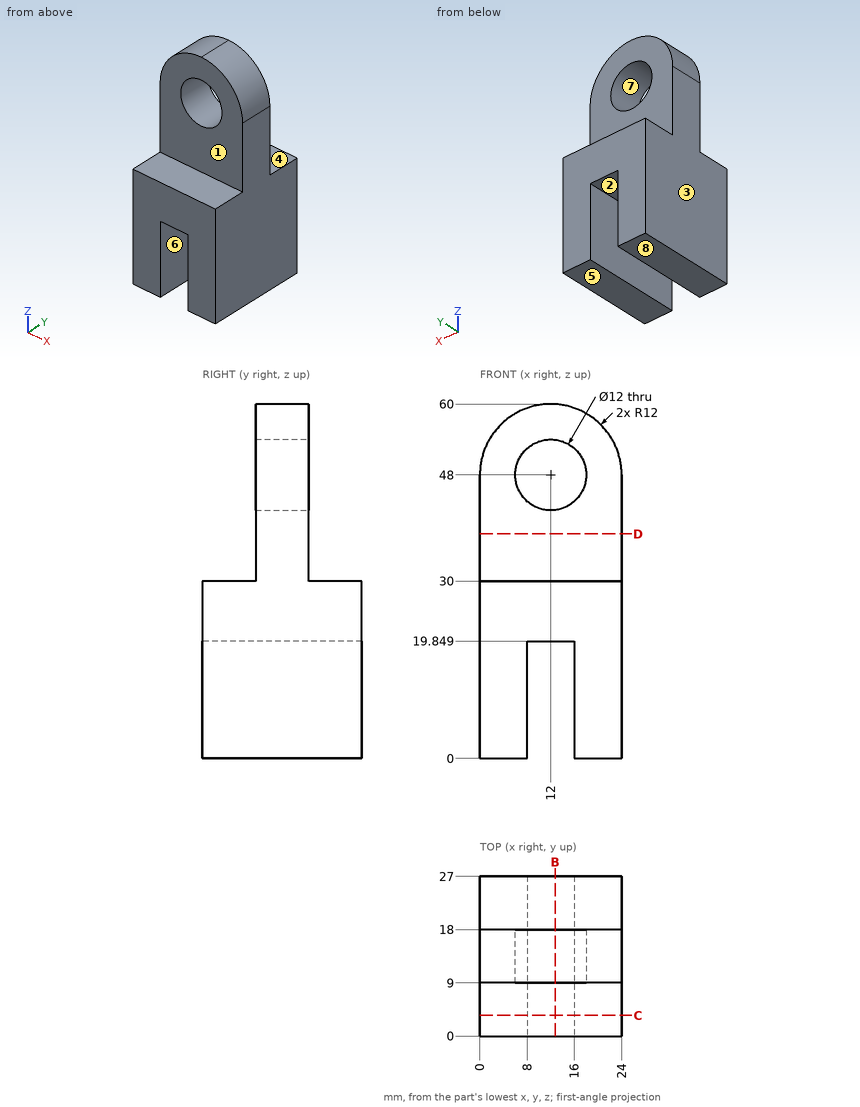
Design review of the part shown in the three views and the two pictorial views. Dimensions are in mm from the part's minimum x, y and z. A direction names the side the tool comes from. Give positions to 0.01 mm unless a question says otherwise; leave off trailing zeros. Write each loop counter-clockwise with the first axis right and the second up, starting at its lowest first coordinate (ties: lowest second). Pieces come first, ordered by that corner, then holes. Notation, with made-up numbers: (29.5, 73.5) -> (37.5, 73.5) arc R23 cw to (37.5, 86.5) -> close; hole circle Ø10 at (47, 35.5). An arc over 180 degrees is marked (long way). Answer in a Markdown table with one row per item.
1) For L1, parallel to Z at x = 12.25, y = 17.75 (1 decimal); L2, parallel to X at y = 12.25, z = 48; L3, parallel to X at y = 16.75, z = 16, list the stretches that pass through material, from the lowest coordinate up. Write a range as [from, to].
Worked answers:
| item | result |
|---|---|
| L1 | [19.8, 42], [54, 60] |
| L2 | [0, 6], [18, 24] |
| L3 | [0, 8], [16, 24] |
2) Mouldability with a two-part tool opening along Z and no side actions: class the marked faces 6, 7 and 8 as +Z half, -Z half, draft (parallel to the pull), parting line (faces both ways), or undercut.
Worked answers:
| item | result |
|---|---|
| face 6 | draft |
| face 7 | undercut |
| face 8 | -Z half |
3) Clearance check with flat-ended pins moving along their axes: P1, Ø2.5, axis at x = 9.5, y = 20.5, coming from the +Z side; P2, Ø2.5, axis at x = 10.5, y = 7.5, coming from the -Z side; P3, Ø7, axis at x = 15, z = 40, coming from the +Y side. State where each tip first meets the part, or that it passes through.
Worked answers:
| item | result |
|---|---|
| P1 | z = 30 |
| P2 | z = 19.85 |
| P3 | y = 18 |
4) Add section B-B on x = 12.75. State the section outline as (y, z) points.
Worked answers:
| item | result |
|---|---|
| outline | (0, 19.85) -> (27, 19.85) -> (27, 30) -> (18, 30) -> (18, 42.05) -> (9, 42.05) -> (9, 30) -> (0, 30) -> close; (9, 53.95) -> (18, 53.95) -> (18, 59.98) -> (9, 59.98) -> close |
5) Tool access review of the marked faces 1, 2, 3, 4 and 5: name each direction out of +Z, -Z, +X, -X, +Y, -Y from which nothing blocks a thin tool from reaching the whole face with its end or side.
Worked answers:
| item | result |
|---|---|
| face 1 | +Z, +X, -X, -Y |
| face 2 | -Z, +Y, -Y |
| face 3 | +Z, -Z, -X, +Y, -Y |
| face 4 | +Z, +X, -X, +Y |
| face 5 | -Z, +X, -X, +Y, -Y |
6) Add section D-D on z = 38. State the section outline as (x, y) points, plus the area to 3 significant figures.
Worked answers:
| item | result |
|---|---|
| outline | (0, 9) -> (24, 9) -> (24, 18) -> (0, 18) -> close |
| area | 216 mm² |
7) Add section C-C on y = 3.5. State the section outline as (x, z) points.
Worked answers:
| item | result |
|---|---|
| outline | (0, 0) -> (8, 0) -> (8, 19.85) -> (16, 19.85) -> (16, 0) -> (24, 0) -> (24, 30) -> (0, 30) -> close |
